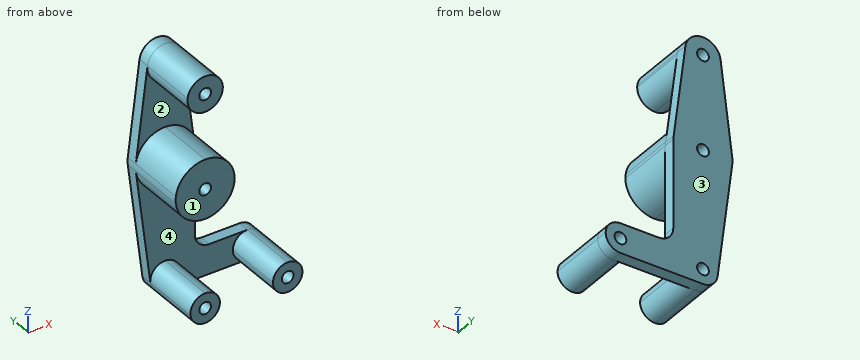
```python
from build123d import *

# Parameters (mm, degrees)
F1_DEPTH = 6.35
F2_DEPTH = 31.75


with BuildPart() as f1:
    # F0 (on Front) → F1 (new body)
    with BuildSketch(Plane.XZ):
        with BuildLine():
            ThreePointArc((0, -15.875), (11.2253201513, -11.2253201513), (15.875, 0))
            ThreePointArc((15.875, 0), (15.8438414983, 0.9941386111), (15.7504883051, 1.9843747505))
            ThreePointArc((15.7504883051, 1.9843747505), (10.5003256101, 11.9062499168), (0, 15.875))
            Line((0, 15.875), (0, 3.175))
            ThreePointArc((0, 3.175), (2.2450640303, 2.2450640303), (3.175, 0))
            ThreePointArc((3.175, 0), (2.2450640303, -2.2450640303), (0, -3.175))
            Line((0, -3.175), (0, -15.875))
        make_face()
        with BuildLine():
            ThreePointArc((-15.7504893995, -1.9843660644), (-10.5003288931, -11.9062470215), (0, -15.875))
            Line((0, -15.875), (0, -3.175))
            ThreePointArc((0, -3.175), (-3.175, 0), (0, 3.175))
            Line((0, 3.175), (0, 15.875))
            ThreePointArc((0, 15.875), (-10.5003288957, 11.9062470192), (-15.7504894003, 1.9843660577))
            ThreePointArc((-15.7504894003, 1.9843660577), (-15.875, -3.4e-09), (-15.7504893995, -1.9843660644))
        make_face()
        with BuildLine():
            ThreePointArc((9.525, 50.8), (9.5063048942, 51.396483242), (9.4502929642, 51.990625))
            ThreePointArc((9.4502929642, 51.990625), (0, 60.325), (-9.4502929642, 51.990625))
            ThreePointArc((-9.4502929642, 51.990625), (-7.14375, 44.4998046905), (0, 41.275))
            ThreePointArc((0, 41.275), (6.7351920908, 44.0648079092), (9.525, 50.8))
        make_face()
        with BuildLine():
            ThreePointArc((3.175, 50.8), (2.2450640303, 48.5549359697), (0, 47.625))
            ThreePointArc((0, 47.625), (-2.2450640303, 53.0450640303), (3.175, 50.8))
        make_face(mode=Mode.SUBTRACT)
        with BuildLine():
            ThreePointArc((7.937499997, -63.5), (5.6126600736, -57.8873399264), (0, -55.562500003))
            Line((0, -55.562500003), (0, -60.325))
            ThreePointArc((0, -60.325), (2.2450640303, -61.2549359697), (3.175, -63.5))
            Line((3.175, -63.5), (7.937499997, -63.5))
        make_face()
        with BuildLine():
            Line((0, -60.325), (0, -55.562500003))
            ThreePointArc((0, -55.562500003), (-5.9531249979, -58.2498372442), (-7.8752441339, -64.4921875))
            ThreePointArc((-7.8752441339, -64.4921875), (-5.2501627558, -69.4531249979), (0, -71.437499997))
            ThreePointArc((0, -71.437499997), (5.6126600736, -69.1126600736), (7.937499997, -63.5))
            Line((7.937499997, -63.5), (3.175, -63.5))
            ThreePointArc((3.175, -63.5), (-2.2450640303, -65.7450640303), (0, -60.325))
        make_face()
        with BuildLine():
            ThreePointArc((44.45, -55.562499997), (38.8373399222, -57.8873399222), (36.512499997, -63.5))
            ThreePointArc((36.512499997, -63.5), (38.8373399222, -69.1126600778), (44.45, -71.437500003))
            ThreePointArc((44.45, -71.437500003), (50.0626600778, -69.1126600778), (52.387500003, -63.5))
            ThreePointArc((52.387500003, -63.5), (50.0626600778, -57.8873399222), (44.45, -55.562499997))
        make_face()
        with BuildLine():
            ThreePointArc((47.625, -63.5), (44.45, -66.675), (41.275, -63.5))
            ThreePointArc((41.275, -63.5), (44.45, -60.325), (47.625, -63.5))
        make_face(mode=Mode.SUBTRACT)
        with BuildLine():
            ThreePointArc((-15.7504894003, 1.9843660577), (-10.5003288957, 11.9062470192), (0, 15.875))
            Line((0, 15.875), (0, 41.275))
            ThreePointArc((0, 41.275), (-7.14375, 44.4998046905), (-9.4502929642, 51.990625))
            Line((-9.4502929642, 51.990625), (-15.7504894003, 1.9843660577))
        make_face()
        with BuildLine():
            ThreePointArc((15.7504883051, 1.9843747505), (15.8438414983, 0.9941386111), (15.875, 0))
            ThreePointArc((15.875, 0), (11.2253201513, -11.2253201513), (0, -15.875))
            Line((0, -15.875), (0, -55.562500003))
            ThreePointArc((0, -55.562500003), (5.6126600736, -57.8873399264), (7.937499997, -63.5))
            Line((7.937499997, -63.5), (36.512499997, -63.5))
            ThreePointArc((36.512499997, -63.5), (38.8373399222, -57.8873399222), (44.45, -55.562499997))
            Line((44.45, -55.5624999909), (23.9506960241, -55.5624999909))
            ThreePointArc((23.9506960241, -55.5624999909), (18.3290556923, -53.2339403227), (16.0004960241, -47.6122999909))
            Line((16.0004960241, -47.6122999909), (16.0004960241, 0))
            Line((16.0004960241, 0), (15.7504883051, 1.9843747505))
        make_face()
        with BuildLine():
            Line((0, -55.562500003), (0, -15.875))
            ThreePointArc((0, -15.875), (-10.5003288931, -11.9062470215), (-15.7504893995, -1.9843660644))
            Line((-15.7504893995, -1.9843660644), (-7.8752441339, -64.4921875))
            ThreePointArc((-7.8752441339, -64.4921875), (-5.9531249979, -58.2498372442), (0, -55.562500003))
        make_face()
        with BuildLine():
            ThreePointArc((0, 15.875), (10.5003256101, 11.9062499168), (15.7504883051, 1.9843747505))
            Line((15.7504883051, 1.9843747505), (9.4502929642, 51.990625))
            ThreePointArc((9.4502929642, 51.990625), (9.5063048942, 51.396483242), (9.525, 50.8))
            ThreePointArc((9.525, 50.8), (6.7351920908, 44.0648079092), (0, 41.275))
            Line((0, 41.275), (0, 15.875))
        make_face()
        with BuildLine():
            Line((36.512499997, -63.5), (7.937499997, -63.5))
            ThreePointArc((7.937499997, -63.5), (5.6126600736, -69.1126600736), (0, -71.437499997))
            Line((0, -71.4374999998), (44.45, -71.4374999998))
            ThreePointArc((44.45, -71.437500003), (38.8373399222, -69.1126600778), (36.512499997, -63.5))
        make_face()
    extrude(amount=-F1_DEPTH)

    # F0 (on Front) → F2 (join)
    with BuildSketch(Plane.XZ):
        with BuildLine():
            ThreePointArc((-15.7504893995, -1.9843660644), (-10.5003288931, -11.9062470215), (0, -15.875))
            Line((0, -15.875), (0, -3.175))
            ThreePointArc((0, -3.175), (-3.175, 0), (0, 3.175))
            Line((0, 3.175), (0, 15.875))
            ThreePointArc((0, 15.875), (-10.5003288957, 11.9062470192), (-15.7504894003, 1.9843660577))
            ThreePointArc((-15.7504894003, 1.9843660577), (-15.875, -3.4e-09), (-15.7504893995, -1.9843660644))
        make_face()
        with BuildLine():
            ThreePointArc((0, -15.875), (11.2253201513, -11.2253201513), (15.875, 0))
            ThreePointArc((15.875, 0), (15.8438414983, 0.9941386111), (15.7504883051, 1.9843747505))
            ThreePointArc((15.7504883051, 1.9843747505), (10.5003256101, 11.9062499168), (0, 15.875))
            Line((0, 15.875), (0, 3.175))
            ThreePointArc((0, 3.175), (2.2450640303, 2.2450640303), (3.175, 0))
            ThreePointArc((3.175, 0), (2.2450640303, -2.2450640303), (0, -3.175))
            Line((0, -3.175), (0, -15.875))
        make_face()
        with BuildLine():
            Line((0, -60.325), (0, -55.562500003))
            ThreePointArc((0, -55.562500003), (-5.9531249979, -58.2498372442), (-7.8752441339, -64.4921875))
            ThreePointArc((-7.8752441339, -64.4921875), (-5.2501627558, -69.4531249979), (0, -71.437499997))
            ThreePointArc((0, -71.437499997), (5.6126600736, -69.1126600736), (7.937499997, -63.5))
            Line((7.937499997, -63.5), (3.175, -63.5))
            ThreePointArc((3.175, -63.5), (-2.2450640303, -65.7450640303), (0, -60.325))
        make_face()
        with BuildLine():
            ThreePointArc((7.937499997, -63.5), (5.6126600736, -57.8873399264), (0, -55.562500003))
            Line((0, -55.562500003), (0, -60.325))
            ThreePointArc((0, -60.325), (2.2450640303, -61.2549359697), (3.175, -63.5))
            Line((3.175, -63.5), (7.937499997, -63.5))
        make_face()
        with BuildLine():
            ThreePointArc((44.45, -55.562499997), (38.8373399222, -57.8873399222), (36.512499997, -63.5))
            ThreePointArc((36.512499997, -63.5), (38.8373399222, -69.1126600778), (44.45, -71.437500003))
            ThreePointArc((44.45, -71.437500003), (50.0626600778, -69.1126600778), (52.387500003, -63.5))
            ThreePointArc((52.387500003, -63.5), (50.0626600778, -57.8873399222), (44.45, -55.562499997))
        make_face()
        with BuildLine():
            ThreePointArc((47.625, -63.5), (44.45, -66.675), (41.275, -63.5))
            ThreePointArc((41.275, -63.5), (44.45, -60.325), (47.625, -63.5))
        make_face(mode=Mode.SUBTRACT)
        with BuildLine():
            ThreePointArc((9.525, 50.8), (9.5063048942, 51.396483242), (9.4502929642, 51.990625))
            ThreePointArc((9.4502929642, 51.990625), (0, 60.325), (-9.4502929642, 51.990625))
            ThreePointArc((-9.4502929642, 51.990625), (-7.14375, 44.4998046905), (0, 41.275))
            ThreePointArc((0, 41.275), (6.7351920908, 44.0648079092), (9.525, 50.8))
        make_face()
        with BuildLine():
            ThreePointArc((3.175, 50.8), (2.2450640303, 48.5549359697), (0, 47.625))
            ThreePointArc((0, 47.625), (-2.2450640303, 53.0450640303), (3.175, 50.8))
        make_face(mode=Mode.SUBTRACT)
    extrude(amount=F2_DEPTH)


solid = f1.part
```
Geometry: final body of the model. Coordinates: model frame, mm. Face numbers are marked on the shaded views. A direction names the side the tool comes from. Coordinates: 2 decimals unless noted, no trailing zeros. Order: outer loops, then holes, each group sorted by start corner. A loop starts at its lowest first (then second) coordinate and runs counter-clockwise, first axis right, second up. Notation, with made-up numbers: (-9, -33.75) -> (41, -33.75) arc R31 cw to (41, -0.75) -> close; hole circle Ø10 at (71, 50.25). An arc over 180 degrees is marked (long way). Write each question's results on one line, items separated by ' | '. Start each with the question number.
1) Cut plane A-A, the plane y = -5.5. State how many separate pieces and enclosed holes the cut face has, and give its area (3 significant figures).
2) Mould query, pull axis Z, two halves, no side actions, for the marked faces 1 and 2. Classes: released by +Z, released by -Z, zero draft, split by the parting line, or undercut.
3) Material intervals for line 1 along X through (y, z) = (4.25, -63.5) (1 decimal); line 2 along X through (y, z) = (-14, -63); line 3 along Y through (x, z) = (5.5, 35), sorted ascending.
4) Set-up query: the marked faces 3 and 4. Return all of +Z, -Z, +X, -X, +Y, -Y with unobstructed straight access to the full face (end or side cutting, diameter ignored); none if empty.
5) Cut plane D-D, the plane z = 22.5. Output: boundary loops of the cut face in (x, y), and give its area (3 significant figures).
6) First-contact query: pin 1 (6 mm diameter, centred on y = -14.5, z = 15.5, fed in from +X); pin 2 (1.5 mm diameter, centred on x = 0.5, z = 40, fed in from -Y); pin 3 (5 mm diameter, centred on x = 34.5, y = 2, fed in from +Z). Flat tips, straight axial feed; report the tip coordinate or a pass-through.
7) Cut plane C-C, the plane x = 5. Output: boundary loops of the cut face in (y, z).
Checks:
1) separate pieces: 4 | enclosed holes: 4 | area: 1,350 mm^2
2) face 1: zero draft | face 2: undercut
3) line 1: -8 to -3.2, 3.2 to 41.3, 47.6 to 52.4 | line 2: -7.92 to -3.14, 3.14 to 7.92, 36.53 to 41.31, 47.59 to 52.37 | line 3: 0 to 6.35
4) face 3: +Z, -Z, +X, -X, +Y | face 4: -Y
5) outline: (-13.17, 0) -> (13.17, 0) -> (13.17, 6.35) -> (-13.17, 6.35) -> close | area: 167 mm^2
6) pin 1: x = 9.79 | pin 2: y = 0 | pin 3: z = -55.56
7) outline: (-31.75, -69.66) -> (0, -69.66) -> (0, -71.44) -> (6.35, -71.44) -> (6.35, 58.91) -> (-31.75, 58.91) -> (-31.75, 42.69) -> (0, 42.69) -> (0, 15.07) -> (-31.75, 15.07) -> (-31.75, -15.07) -> (0, -15.07) -> (0, -57.34) -> (-31.75, -57.34) -> close
